Here's how the part is built. I have some questions about the finished solid (model axes, mm). Face numbers are marked on the shaded views. A direction names the side the tool comes from. Round coordinates to 2 decimals unless told otherwise and drop trailing zeros. Write each loop counter-clockwise with the first axis right and the second up, starting at its lowest first coordinate (ties: lowest second). Pieces come first, ordered by that corner, then holes. Notation, with made-up numbers: (36.25, 43) -> (40.25, 43) arc R34 ccw to (40.25, 80) -> close; hole circle Ø8 at (45, 33.5). An arc over 180 degrees is marked (long way). Put each result on its own line as item: value. Start each with the question number.
1) I want a section at C-C, the plane z = 1. List the corners of the cut face in (x, y) for me.
2) I want a section at D-D, the plane y = -7. List the corners of the cut face in (x, z) for me (3 decimals), then the cut area to 3 significant figures.
3) Which directions (+Z, -Z, +X, -X, +Y, -Y) give clear straight access to the entire face, cutting with the end or side of a thin tool? Please do the marked faces 1, 2 and 3.
4) I want a section at A-A, the plane y = -14.5. List the corners of the cut face in (x, z) for me, then the cut area to 3 significant figures.
5) I want a section at B-B, the plane x = 0. List the corners of the cut face in (y, z) for me, then the cut area to 3 significant figures.
6) If I drill on line 1 along X through (y, z) = (-11, 0.5); line 2 along Y through (x, z) = (12, 1); line 3 along Y through (x, z) = (2, -9), over which ranges is the centre line in solid material (lowest first)? Write a range as [from, to].
7) Will these pins go through, and if not, where does the flat tip stop? P1, Ø13, axis at x = 8, y = -6.5, coming from the -Z side; P2, Ø2.5, axis at x = -2.5, z = -8, coming from the +Y side; P3, Ø8, axis at x = -6.5, y = -4.5, coming from the +Z side; P4, Ø10, axis at y = -42, z = -5.5, coming from the +X side.
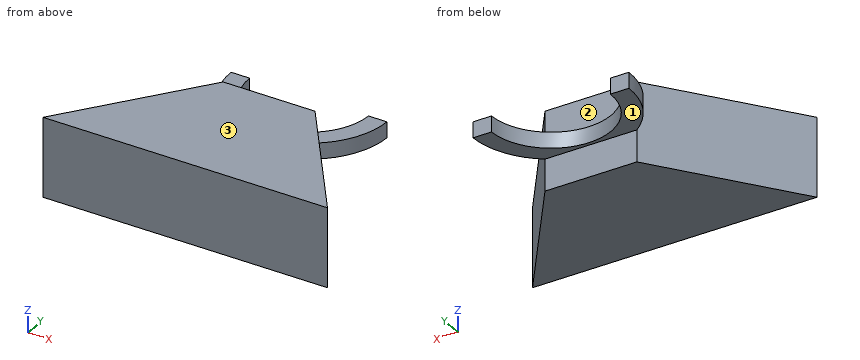
from build123d import *

# Parameters (mm, degrees)
BOSS_EXTRU_1_DEPTH      = 2
BOSS_EXTRU_1_DEPTH_BACK = 2
BOSS_EXTRU_3_DEPTH      = 10
BOSS_EXTRU_3_DEPTH_BACK = 10


with BuildPart() as part:
    # Esquisse1 → Boss.-Extru.1 (new, two sides: drawn at the far end of the back side and taken through both)
    with BuildSketch(Plane.XY.offset(-BOSS_EXTRU_1_DEPTH_BACK)):
        with BuildLine():
            Line((-20, 0), (-15.25, 0))
            ThreePointArc((-15.25, 0), (0, -15.25), (15.25, 0))
            Line((15.25, 0), (20, 0))
            ThreePointArc((20, 0), (0, -20), (-20, 0))
        make_face()
    extrude(amount=BOSS_EXTRU_1_DEPTH + BOSS_EXTRU_1_DEPTH_BACK)

    # Esquisse2 → Boss.-Extru.3 (add, two sides: drawn at the far end of the back side and taken through both)
    with BuildSketch(Plane.XY.offset(-BOSS_EXTRU_3_DEPTH_BACK)):
        Polygon((-36.508808232, -50), (-11.79408626, -16.152384632), (11.79408626, -16.152384632), (36.508808232, -50), align=None)
    extrude(amount=BOSS_EXTRU_3_DEPTH + BOSS_EXTRU_3_DEPTH_BACK)


solid = part.part
Findings:
1. outline: (-36.51, -50) -> (36.51, -50) -> (11.79, -16.15) arc R20 ccw to (20, 0) -> (15.25, 0) arc R15.25 cw to (-15.25, 0) -> (-20, 0) arc R20 ccw to (-11.79, -16.15) -> close
2. outline: (-18.735, -2) -> (-13.549, -2) -> (-13.549, 2) -> (-18.735, 2) -> close; (13.549, -2) -> (18.735, -2) -> (18.735, 2) -> (13.549, 2) -> close
2. area: 41.5 mm2
3. face 1: -Z, +X, -X, +Y
3. face 2: +Z, +X, -X, +Y
3. face 3: +Z, +X, -X, +Y, -Y
4. outline: (-13.77, -2) -> (-4.72, -2) -> (-4.72, 2) -> (-13.77, 2) -> close; (4.72, -2) -> (13.77, -2) -> (13.77, 2) -> (4.72, 2) -> close
4. area: 72.4 mm2
5. outline: (-50, -10) -> (-16.15, -10) -> (-16.15, -2) -> (-15.25, -2) -> (-15.25, 2) -> (-16.15, 2) -> (-16.15, 10) -> (-50, 10) -> close
5. area: 681 mm2
6. line 1: x = [-16.7, -10.56], [10.56, 16.7]
6. line 2: y = [-50, -16.43], [-16, -9.41]
6. line 3: y = [-50, -16.15]
7. P1: stops at z = -2
7. P2: stops at y = -16.15
7. P3: passes through
7. P4: stops at x = 34.32
